Drawing for the job (mm, zero at the part's lowest x, y, z). A direction names the side the tool comes from. Round coordinates to 2 decimals unless told otherwise and drop trailing zeros. Loops run counter-clockwise (first coordinate to the right, second up) from the corner with the lowest first, then second, coordinate; pieces in that order, holes last. Notation, with made-up numbers: (50.5, 28.25) - (93.5, 28.25) arc R38 ccw to (93.5, 66.25) - close; hole circle Ø6 at (28.25, 3.5). An arc over 180 degrees is marked (long way). Put each result on its own line as item: value.
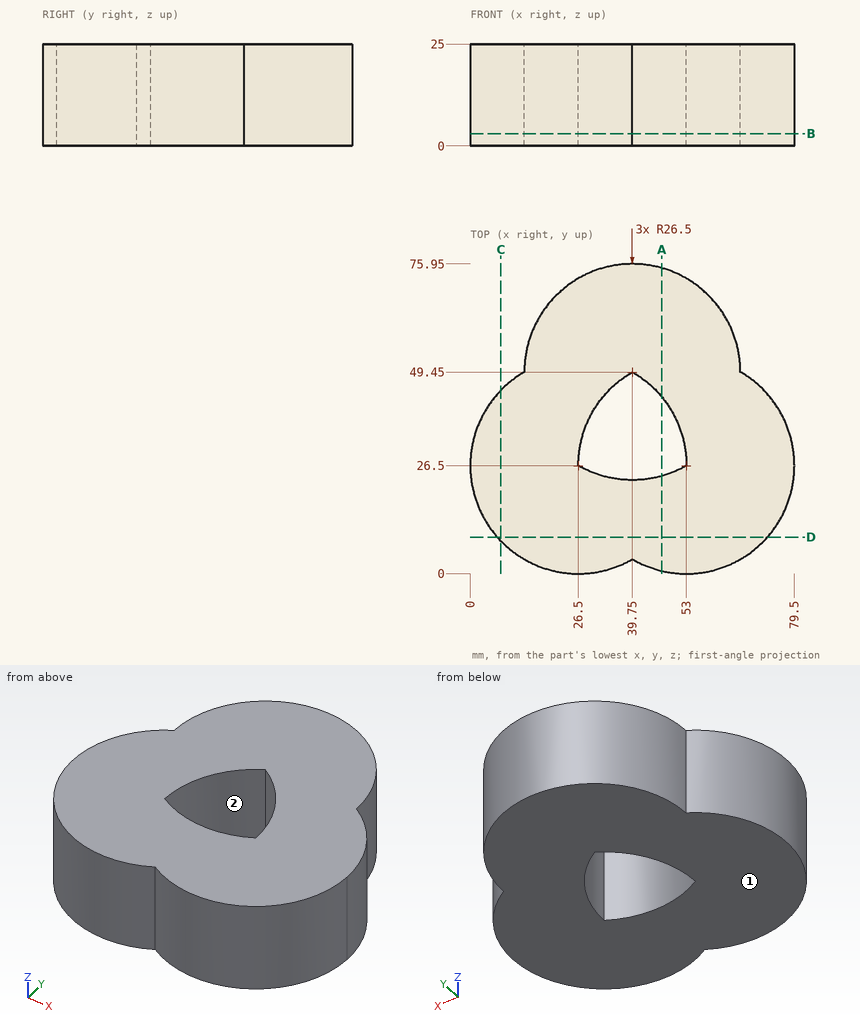
1. Probe line 1 along X through (y, z) = (38, 7.25) (1 decimal); line 2 along X through (y, z) = (26, 21) (1 decimal); line 3 along Y through (x, z) = (42.5, 13) (1 decimal). List the from-to ranges inside material, lowest first. Write a range as [from, to].
A:
line 1: x = [2.6, 29.1], [50.4, 76.9]
line 2: x = [0, 27.4], [52.1, 79.5]
line 3: y = [2.2, 23.1], [47.6, 75.8]
2. Pin check, flat tips, straight feed: P1, Ø1.5, axis at x = 23.5, z = 10.5, coming from the -Y side; P2, Ø12, axis at x = 52.5, z = 13.5, coming from the +Y side (1 decimal); P3, Ø1.5, axis at x = 57, z = 14.5, coming from the +Y side (1 decimal). Stop position of each tip, or through.
A:
P1: stops at y = 0.1
P2: stops at y = 75.1
P3: stops at y = 70.2
3. Band-saw the part on B-B (z = 3). List the corners of the cut face in (x, y), plus the area to 3 significant figures.
A:
outline: (13.25, 49.45) arc R26.5 ccw to (39.75, 3.55) arc R26.5 ccw to (66.25, 49.45) arc R26.5 ccw to start; hole (26.5, 26.5) arc R26.5 ccw to (53, 26.5) arc R26.5 ccw to (39.75, 49.45) arc R26.5 ccw to start
area: 4,030 mm²
4. Tool access for the marked faces 1 and 2: list every direction of +Z, -Z, +X, -X, +Y, -Y with a clear straight run to the whole face (end or side of a thin tool).
A:
face 1: -Z, +X, -X, +Y, -Y
face 2: +Z, -Z
5. Band-saw the part on A-A (x = 47). List the corners of the cut face in (y, z), plus the area to 3 significant figures.
A:
outline: (0.69, 0) - (23.96, 0) - (23.96, 25) - (0.69, 25) - close; (43.29, 0) - (74.94, 0) - (74.94, 25) - (43.29, 25) - close
area: 1,370 mm²
6. Band-saw the part on C-C (x = 7.5). List the corners of the cut face in (y, z), plus the area to 3 significant figures.
A:
outline: (8.03, 0) - (44.97, 0) - (44.97, 25) - (8.03, 25) - close
area: 924 mm²
7. Band-saw the part on D-D (y = 9). List the corners of the cut face in (x, z), plus the area to 3 significant figures.
A:
outline: (6.6, 0) - (72.9, 0) - (72.9, 25) - (6.6, 25) - close
area: 1,660 mm²
